For this review, take the finished solid that the model builds, in its own axes (mm). A direction names the side the tool comes from. Round coordinates to 2 decimals unless told otherwise and drop trailing zeros. Order: outer loops, then holes, each group sorted by start corner. A loop starts at its lowest first (then second) coordinate and runs counter-clockwise, first axis right, second up. Notation, with made-up numbers: M 51,-22 L 75,-22 A29 ccw 75,16 Z; hole C 10,-32.75 d7. An arc over 180 degrees is marked long. Write item = value, one per line. Start each with the question number.
from build123d import *

# Parameters (mm, degrees)
F0_R           = 20
F1_DEPTH       = 270
F4_D           = 17.5
F4_DEPTH       = 52.5
F4_TIP         = 5.2575304165
F4_ON_F3_D     = 17.5
F4_ON_F3_DEPTH = 52.5
F4_ON_F3_TIP   = 5.2575304165


with BuildPart() as f1:
    # F0 (on Right) → F1 (new body, symmetric)
    with BuildSketch(Plane.YZ):
        Circle(F0_R)
    extrude(amount=F1_DEPTH, both=True)

    # F4
    with Locations(Plane.YZ.offset(270)):
        with Locations((0, 0)):
            Hole(F4_D / 2, depth=F4_DEPTH)
            with Locations((0, 0, -(F4_DEPTH + F4_TIP / 2))):  # 118° drill point
                Cone(0, F4_D / 2, F4_TIP, mode=Mode.SUBTRACT)

    # F4 on F3
    with Locations(Plane(origin=(-270, 0, 0), x_dir=(0, -1, 0), z_dir=(-1, 0, 0))):
        with Locations((0, 0)):
            Hole(F4_ON_F3_D / 2, depth=F4_ON_F3_DEPTH)
            with Locations((0, 0, -(F4_ON_F3_DEPTH + F4_ON_F3_TIP / 2))):  # 118° drill point
                Cone(0, F4_ON_F3_D / 2, F4_ON_F3_TIP, mode=Mode.SUBTRACT)


solid = f1.part
(1) For line 1 along Z through (x, y) = (255, 0); line 2 along Y through (x, z) = (-246, 1); line 3 along Z through (x, y) = (131.5, 0), list the stretches that pass through material, from the lowest coordinate up.
(2) We need section A-A, the plane x = -26.5. Write out the cut boundary in (y, z), then the cut area to 3 significant figures.
(3) Insertion check: pin 1 (12 mm diameter, centred on x = 100, y = -1.5, fed in from +Z); pin 2 (2 mm diameter, centred on x = -116.5, y = -8.5, fed in from -Z); pin 3 (2 mm diameter, centred on x = -135.5, y = 12.5, fed in from +Z). Each pin has a flat end and moves straight along its axis. Give the tip position at first contact, or say it passes through.
(4) Draft analysis for pull direction Y (two halves, no side actions). For faces 4 (the conical face through (-213.156, 0.329, -1.483)), 5 (the cylindrical face through (3.78, -4.336, -19.524)), 6 (the flat face through (270, 9, -4)), state which applies: released by +Y, released by -Y, zero draft, split by the parting line, or undercut.
(5) For faces 1 (the flat face through (-270, 9, -4)), 2 (the cylindrical face through (-243.382, -6.944, -5.324)), 3 (the cylindrical face through (243.382, 6.944, -5.324)), list the 3-axis set-ups (+Z, -Z, +X, -X, +Y, -Y) from which the entire face can be reached by the end or side of a thin tool; tool diameter is ignored.
(6) We need section B-B, the plane y = -15.5. Write out the cut boundary in (x, z).
Values:
q1.line_1 = -20 to -8.75, 8.75 to 20
q1.line_2 = -19.97 to -8.69, 8.69 to 19.97
q1.line_3 = -20 to 20
q2.outline = C 0,0 d40
q2.area = 1,260 mm²
q3.pin_1 = 20
q3.pin_2 = -18.54
q3.pin_3 = 16.36
q4.face_4 = undercut
q4.face_5 = split by the parting line
q4.face_6 = zero draft
q5.face_1 = +Z, -Z, -X, +Y, -Y
q5.face_2 = -X
q5.face_3 = +X
q6.outline = M -270,-12.64 L 270,-12.64 L 270,12.64 L -270,12.64 Z
